from build123d import *

# Parameters (mm, degrees)
SKETCH1_W           = 90
SKETCH1_H           = 30
SKETCH1_R           = 9
BOSS_EXTRUDE1_DEPTH = 5
SKETCH2_W           = 30
SKETCH2_H           = 30
BOSS_EXTRUDE2_DEPTH = 1
SKETCH3_W           = 30
SKETCH3_H           = 30
BOSS_EXTRUDE3_DEPTH = 2
SKETCH4_W           = 30
SKETCH4_H           = 30
BOSS_EXTRUDE4_DEPTH = 3
SKETCH5_W           = 30
SKETCH5_H           = 30
SKETCH5_R           = 12.75
BOSS_EXTRUDE5_DEPTH = 10
SKETCH6_W           = 30
SKETCH6_H           = 30
SKETCH6_R           = 12.75
BOSS_EXTRUDE6_DEPTH = 10
SKETCH7_W           = 30
SKETCH7_H           = 30
SKETCH7_R           = 12.75
BOSS_EXTRUDE7_DEPTH = 10


with BuildPart() as part:
    # Sketch1 → Boss-Extrude1 (new body)
    with BuildSketch(Plane(origin=(0, 0, 0), x_dir=(1, 0, 0), z_dir=(0, 1, 0))):
        Rectangle(SKETCH1_W, SKETCH1_H)
        with Locations(Location((-30, 0, 0), (0, 0, 270))):
            Circle(SKETCH1_R, mode=Mode.SUBTRACT)
        with Locations(Location((0, 0, 0), (0, 0, 270))):
            Circle(SKETCH1_R, mode=Mode.SUBTRACT)
        with Locations(Location((30, 0, 0), (0, 0, 270))):
            Circle(SKETCH1_R, mode=Mode.SUBTRACT)
    extrude(amount=BOSS_EXTRUDE1_DEPTH)

    # Sketch2 → Boss-Extrude2 (add)
    with BuildSketch(Plane(origin=(0, 5, 0), x_dir=(1, 0, 0), z_dir=(0, 1, 0))):
        with Locations((-30, 0)):
            Rectangle(SKETCH2_W, SKETCH2_H)
    extrude(amount=BOSS_EXTRUDE2_DEPTH)

    # Sketch3 → Boss-Extrude3 (add)
    with BuildSketch(Plane(origin=(0, 5, 0), x_dir=(1, 0, 0), z_dir=(0, 1, 0))):
        Rectangle(SKETCH3_W, SKETCH3_H)
    extrude(amount=BOSS_EXTRUDE3_DEPTH)

    # Sketch4 → Boss-Extrude4 (add)
    with BuildSketch(Plane(origin=(0, 5, 0), x_dir=(1, 0, 0), z_dir=(0, 1, 0))):
        with Locations((30, 0)):
            Rectangle(SKETCH4_W, SKETCH4_H)
    extrude(amount=BOSS_EXTRUDE4_DEPTH)

    # Sketch5 → Boss-Extrude5 (add)
    with BuildSketch(Plane(origin=(0, 6, 0), x_dir=(1, 0, 0), z_dir=(0, 1, 0))):
        with Locations((-30, 0)):
            Rectangle(SKETCH5_W, SKETCH5_H)
        with Locations(Location((-30, 0, 0), (0, 0, 270))):
            Circle(SKETCH5_R, mode=Mode.SUBTRACT)
    extrude(amount=BOSS_EXTRUDE5_DEPTH)

    # Sketch6 → Boss-Extrude6 (add)
    with BuildSketch(Plane(origin=(0, 7, 0), x_dir=(1, 0, 0), z_dir=(0, 1, 0))):
        Rectangle(SKETCH6_W, SKETCH6_H)
        with Locations(Location((0, 0, 0), (0, 0, 270))):
            Circle(SKETCH6_R, mode=Mode.SUBTRACT)
    extrude(amount=BOSS_EXTRUDE6_DEPTH)

    # Sketch7 → Boss-Extrude7 (add)
    with BuildSketch(Plane(origin=(0, 8, 0), x_dir=(1, 0, 0), z_dir=(0, 1, 0))):
        with Locations((30, 0)):
            Rectangle(SKETCH7_W, SKETCH7_H)
        with Locations(Location((30, 0, 0), (0, 0, 270))):
            Circle(SKETCH7_R, mode=Mode.SUBTRACT)
    extrude(amount=BOSS_EXTRUDE7_DEPTH)


solid = part.part
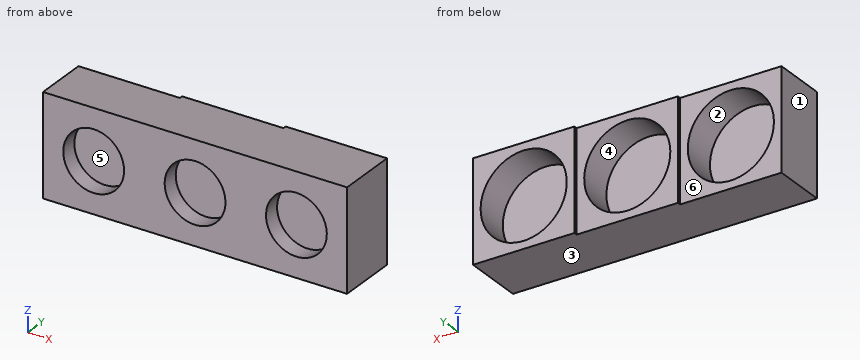
Input: part model. Units: mm. Frame: model coordinates. Face numbers are marked on the shaded views. A direction names the side the tool comes from. Coordinates: 2 decimals unless noted, no trailing zeros. Loops run counter-clockwise (first coordinate to the right, second up) from the corner with the lowest first, then second, coordinate; pieces in that order, holes last. Notation, with made-up numbers: (-2.75, 60.5) - (5.25, 60.5) arc R20 ccw to (5.25, 84.5) - close; hole circle Ø11 at (20.25, 39). An arc over 180 degrees is marked (long way). Answer in a Markdown table with one row per item. Add a question column.
Item 1: Mould query, pull axis Z, two halves, no side actions, for the marked faces 1, 2 and 3. Classes: released by +Z, released by -Z, zero draft, split by the parting line, or undercut.
Item 2: Section query A-A on y = 3.25. Return the cut outline in (x, z), then the cut area to 3 significant figures.
Item 3: Section query B-B on x = -30. Return the cut outline in (y, z).
Item 4: Line query: line 1 along X through (y, z) = (13.5, 0); line 2 along X through (y, z) = (1.6, 0); line 3 along X through (y, z) = (7.5, 10.5). Output: solid intervals per line, ascending. Write a range as [from, to].
Item 5: Section query D-D on y = 14.5. Return the cut outline in (x, z).
Item 6: Access query for the marked faces 4, 5 and 6. Directions: +Z, -Z, +X, -X, +Y, -Y. A direction counts if a zero-diameter tool reaches every point of the face in a straight line with its end or side. Return the directions, or none.
Item 7: Contact query for flat-ended pins moving along their axis: P1, Ø8, axis at x = 28.5, z = 4, coming from the +Y side; P2, Ø9, axis at x = 28, z = -3.5, coming from the -Y side; P3, Ø13, axis at x = -32, z = 4, coming from the +Y side. Output: stop coordinate, or through.
Recorded:
| question | item | result |
|---|---|---|
| 1 | face 1 | zero draft |
| 1 | face 2 | undercut |
| 1 | face 3 | released by -Z |
| 2 | outline | (-45, -15) - (45, -15) - (45, 15) - (-45, 15) - close; hole circle Ø18 at (-30, 0); hole circle Ø18 at (0, 0); hole circle Ø18 at (30, 0) |
| 2 | area | 1,940 mm^2 |
| 3 | outline | (0, -15) - (16, -15) - (16, -12.75) - (6, -12.75) - (6, 12.75) - (16, 12.75) - (16, 15) - (0, 15) - (0, 9) - (5, 9) - (5, -9) - (0, -9) - close |
| 4 | line 1 | [-45, -42.75], [-17.25, -12.75], [12.75, 17.25], [42.75, 45] |
| 4 | line 2 | [-45, -39], [-21, -9], [9, 21], [39, 45] |
| 4 | line 3 | [-45, -37.23], [-22.77, -7.23], [7.23, 45] |
| 5 | outline | (-45, -15) - (45, -15) - (45, 15) - (-45, 15) - close; hole circle Ø25.5 at (-30, 0); hole circle Ø25.5 at (0, 0); hole circle Ø25.5 at (30, 0) |
| 6 | face 4 | +Y |
| 6 | face 5 | -Y |
| 6 | face 6 | +Z, -Z, -X, +Y |
| 7 | P1 | y = 8 |
| 7 | P2 | y = 5 |
| 7 | P3 | y = 6 |
